Design review of the part built by this model. Coordinates are the model's own, in mm. Face numbers are marked on the shaded views. A direction names the side the tool comes from. Give positions to 0.01 mm unless a question says otherwise; leave off trailing zeros. Order: outer loops, then holes, each group sorted by start corner. A loop starts at its lowest first (then second) coordinate and runs counter-clockwise, first axis right, second up. Notation, with made-up numbers: (60.25, 77) -> (74.25, 77) arc R33 cw to (74.25, 113) -> close; hole circle Ø4 at (83, 17.5). An arc over 180 degrees is marked (long way). Return JSON: item names as keys, results as strings.
```python
from build123d import *

# Parameters (mm, degrees)
SKETCH5_W                       = 176
SKETCH5_H                       = 90
SKETCH5_W_2                     = 161
SKETCH5_H_2                     = 80.5
BOSS_EXTRUDE2_DEPTH             = 25
M4X0_7_TAPPED_HOLE1_D           = 3.3
CBORE_FOR_M4_SBHCS1_D           = 4.5
CBORE_FOR_M4_SBHCS1_DEPTH       = 4.75
CBORE_FOR_M4_SBHCS1_CBORE_D     = 8.6
CBORE_FOR_M4_SBHCS1_CBORE_DEPTH = 2.75
M4X0_7_TAPPED_HOLE2_D           = 3.3
M4X0_7_TAPPED_HOLE2_DEPTH       = 5
M4X0_7_TAPPED_HOLE2_TIP         = 0.991420021


with BuildPart() as part:
    # Sketch5 → Boss-Extrude2 (new body)
    with BuildSketch(Plane.XY):
        Rectangle(SKETCH5_W, SKETCH5_H)
        Rectangle(SKETCH5_W_2, SKETCH5_H_2, mode=Mode.SUBTRACT)
    extrude(amount=BOSS_EXTRUDE2_DEPTH)

    # M4x0.7 Tapped Hole1 (through all)
    with Locations(Plane(origin=(0, 0, 0), x_dir=(-1, 0, 0), z_dir=(0, 0, -1))):
        with Locations((0, 0), (84, 40), (-84, -40), (-84, 40), (84, -40)):
            Hole(M4X0_7_TAPPED_HOLE1_D / 2)

    # CBORE for M4 SBHCS1
    with Locations(Plane(origin=(0, -40.25, 0), x_dir=(1, 0, 0), z_dir=(0, 1, 0))):
        with Locations((-60, -15), (60, -15)):
            CounterBoreHole(CBORE_FOR_M4_SBHCS1_D / 2, CBORE_FOR_M4_SBHCS1_CBORE_D / 2, CBORE_FOR_M4_SBHCS1_CBORE_DEPTH, depth=CBORE_FOR_M4_SBHCS1_DEPTH)

    # M4x0.7 Tapped Hole2
    with Locations(Plane(origin=(0, 0, 0), x_dir=(-1, 0, 0), z_dir=(0, 0, -1))):
        with Locations((0, 0), (10, 42.5), (-10, -42.5), (-10, 42.5), (10, -42.5)):
            Hole(M4X0_7_TAPPED_HOLE2_D / 2, depth=M4X0_7_TAPPED_HOLE2_DEPTH)
            with Locations((0, 0, -(M4X0_7_TAPPED_HOLE2_DEPTH + M4X0_7_TAPPED_HOLE2_TIP / 2))):  # 118° drill point
                Cone(0, M4X0_7_TAPPED_HOLE2_D / 2, M4X0_7_TAPPED_HOLE2_TIP, mode=Mode.SUBTRACT)


solid = part.part
```
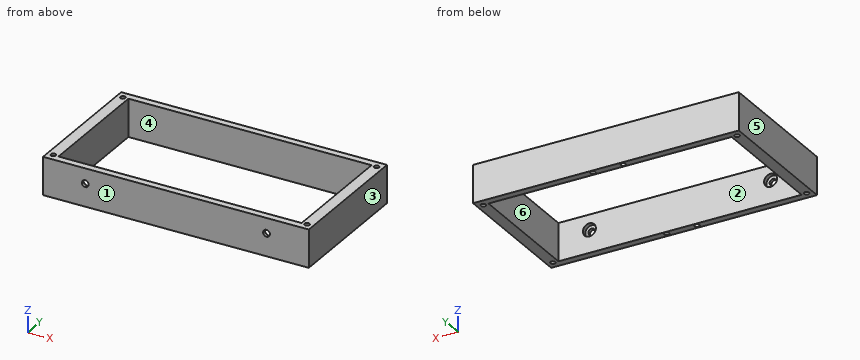
Item 1: Add section D-D (x = -60). Give the boundary of the cut face in (y, z).
Result set:
{"outline": "(-45, 0) -> (-40.25, 0) -> (-40.25, 10.7) -> (-43, 10.7) -> (-43, 12.75) -> (-45, 12.75) -> close; (-45, 17.25) -> (-43, 17.25) -> (-43, 19.3) -> (-40.25, 19.3) -> (-40.25, 25) -> (-45, 25) -> close; (40.25, 0) -> (45, 0) -> (45, 25) -> (40.25, 25) -> close"}
Item 2: Add section A-A (x = -32.5). Give the boundary of the cut face in (y, z).
Result set:
{"outline": "(-45, 0) -> (-40.25, 0) -> (-40.25, 25) -> (-45, 25) -> close; (40.25, 0) -> (45, 0) -> (45, 25) -> (40.25, 25) -> close"}
Item 3: Wall thickness on L1, parallel to Y at x = 84, z = 14.5; L2, parallel to Y at x = -10, z = 1.55; L3, parallel to X at y = 42.5, z = 2.7: over which ranges is each line inside the solid? List them lowest first. Write a range as [from, to].
Result set:
{"L1": "y = [-45, -41.65], [-38.35, 38.35], [41.65, 45]", "L2": "y = [-45, -44.15], [-40.85, -40.25], [40.25, 40.85], [44.15, 45]", "L3": "x = [-88, -11.65], [-8.35, 8.35], [11.65, 88]"}
Item 4: For pin 1 (2.5 mm diameter, centred on x = -84, y = -40, fed in from -Z); pin 2 (3.5 mm diameter, centred on x = -60, z = 15, fed in from -Y); pin 3 (2.5 mm diameter, centred on x = -10, y = 42.5, fed in from -Z), all flat-tipped, find the tip position at first contact; note any pin that passes through.
Result set:
{"pin 1": "passes through", "pin 2": "stops at y = 40.25", "pin 3": "stops at z = 5.24"}
Item 5: Mouldability with a two-part tool opening along X and no side actions: class the marked faces 3, 4, 5 and 6 as released by +X, released by -X, zero draft, split by the parting line, or undercut.
Result set:
{"face 3": "released by +X", "face 4": "undercut", "face 5": "released by -X", "face 6": "undercut"}
Item 6: Add section C-C (z = 22.5). Give the boundary of the cut face in (x, y), plus the area to 3 significant figures.
Result set:
{"outline": "(-88, -45) -> (88, -45) -> (88, 45) -> (-88, 45) -> close; hole circle Ø3.3 at (-84, -40); hole circle Ø3.3 at (-84, 40); hole (-80.5, -40.25) -> (80.5, -40.25) -> (80.5, 40.25) -> (-80.5, 40.25) -> close; hole circle Ø3.3 at (84, -40); hole circle Ø3.3 at (84, 40)", "area": "2,850 mm^2"}
Item 7: Add section B-B (y = 3.5). Give the boundary of the cut face in (x, z).
Result set:
{"outline": "(-88, 0) -> (-80.5, 0) -> (-80.5, 25) -> (-88, 25) -> close; (80.5, 0) -> (88, 0) -> (88, 25) -> (80.5, 25) -> close"}
Item 8: Machinability: for the marked faces 1 and 2, which of the approach directions +Z, -Z, +X, -X, +Y, -Y give a long, thin tool a straight path to every point of the face, cutting with its end or side? Answer none if there is none.
Result set:
{"face 1": "+Z, -Z, +X, -X, -Y", "face 2": "+Z, -Z"}
